Here's how the part is built. I have some questions about the finished solid (model axes, mm). Round coordinates to 2 decimals unless told otherwise and drop trailing zeros. Loops run counter-clockwise (first coordinate to the right, second up) from the corner with the lowest first, then second, coordinate; pieces in that order, holes last. Notation, with made-up numbers: M -32,-16.5 L 27,-16.5 A16 cw 27,8.5 Z; hole C 21.5,42 d3. An arc over 180 degrees is marked long. Answer as a JSON object with one key per item and string values.
from build123d import *

# Parameters (mm, degrees)
DODANIE_WYCI_GNI_CIE1_DEPTH = 12.065
WYTNIJ_WYCI_GNI_CIE1_DEPTH  = 50.230978306


with BuildPart() as part:
    # Szkic1 → Dodanie-wyciągnięcie1 (new, symmetric)
    with BuildSketch(Plane.XY):
        with BuildLine():
            Line((33.75, 0), (31.75, 0))
            ThreePointArc((31.75, 0), (0, 31.75), (-31.75, 0))
            Line((-31.75, 0), (-33.75, 0))
            ThreePointArc((-33.75, 0), (0, 33.75), (33.75, 0))
        make_face()
    extrude(amount=DODANIE_WYCI_GNI_CIE1_DEPTH, both=True)

    # Szkic2 → Wytnij-wyciągnięcie1 (cut, through all)
    with BuildSketch(Plane(origin=(0, 0, 0), x_dir=(-1, 0, 0), z_dir=(0, -1, 0))):
        with BuildLine():
            Line((-33.75, 5.567764363), (-33.75, 0))
            Line((-33.75, 0), (-33.75, -5.567764363))
            ThreePointArc((-33.75, -5.567764363), (-32.75, 0), (-33.75, 5.567764363))
        make_face()
    wytnij_wyci_gni_cie1 = extrude(amount=-WYTNIJ_WYCI_GNI_CIE1_DEPTH, mode=Mode.SUBTRACT)

    # Lustro1: Wytnij-wyciągnięcie1 across plane
    add(wytnij_wyci_gni_cie1.mirror(Plane(origin=(0, 0, 0), x_dir=(0, 0, 1), z_dir=(1, 0, 0))), mode=Mode.SUBTRACT)


solid = part.part
Item 1: Please list where these lines run through material, in increasing order: probe 1 along X at (y, z) = (10, -1); probe 2 along X at (y, z) = (23, -7); probe 3 along Y at (x, z) = (-22, 8.5). Write a range as from..to.
Resolved:
{"probe 1": "-32.23..-30.13, 30.13..32.23", "probe 2": "-24.7..-21.89, 21.89..24.7", "probe 3": "22.89..25.59"}
Item 2: I want a section at C-C, the plane x = 0. Please give me the cut outline in (y, z) (3 decimals).
Resolved:
{"outline": "M 31.75,-12.065 L 33.75,-12.065 L 33.75,12.065 L 31.75,12.065 Z"}
Item 3: If we mould it in two halves opening along X, with no side actions, what happens to faces 1 (the face through (0.698, 31.742, 0.169)), 2 (the face through (32.75, 3.11, 0.08)), 3 (the face through (-32.5, 0, 0.2)), 4 (the face through (-32.75, 3.11, 0.08))? For each: pulls with the +X half, pulls with the -X half, needs draft (parallel to the pull), parting line crosses it, or undercut.
Resolved:
{"face 1": "undercut", "face 2": "pulls with the +X half", "face 3": "needs draft", "face 4": "pulls with the -X half"}
Item 4: I want a section at D-D, the plane y = 24. Please give me the cut outline in (x, z) (3 decimals).
Resolved:
{"outline": "M -23.729,-12.065 L -20.786,-12.065 L -20.786,12.065 L -23.729,12.065 Z; M 20.786,-12.065 L 23.729,-12.065 L 23.729,12.065 L 20.786,12.065 Z"}
Item 5: I want a section at B-B, the plane z = 9. Please give me the cut outline in (x, y).
Resolved:
{"outline": "M -33.75,0 L -31.75,0 A31.75 cw 31.75,0 L 33.75,0 A33.75 ccw Z"}
Item 6: I'm going to push flat-ended pins straight in: pin 1 Ø1 at (y, z) = (30, 6) entering from -X; pin 2 Ø8 at (y, z) = (6, -6) entering from +X; pin 3 Ø12 at (x, z) = (5, 3.5) entering from +Y; pin 4 Ø6 at (x, y) = (24.5, 29.5) entering from -Z. Where does each tip first touch, or does it pass through?
Resolved:
{"pin 1": "x = -16.4", "pin 2": "x = 33.69", "pin 3": "y = 33.75", "pin 4": "through"}
Item 7: I want a section at A-A, the plane y = 28. Please give me the cut outline in (x, z) (3 decimals).
Resolved:
{"outline": "M -18.843,-12.065 L -14.969,-12.065 L -14.969,12.065 L -18.843,12.065 Z; M 14.969,-12.065 L 18.843,-12.065 L 18.843,12.065 L 14.969,12.065 Z"}
